Check sheet for the drawn part. Datum: minimum x, y, z corner. Units: mm. Give positions to 0.01 mm unless a question says otherwise; leave off trailing zeros. Loops run counter-clockwise (first coordinate to the right, second up) from the corner with the lowest first, then second, coordinate; pieces in that order, holes last. Notation, with made-up numbers: (-4, 48.25) - (20, 48.25) arc R22 ccw to (20, 64.25) - close; hole circle Ø10 at (0.5, 72.5). An arc over 180 degrees is marked (long way). Answer in a Markdown table with one row per item.
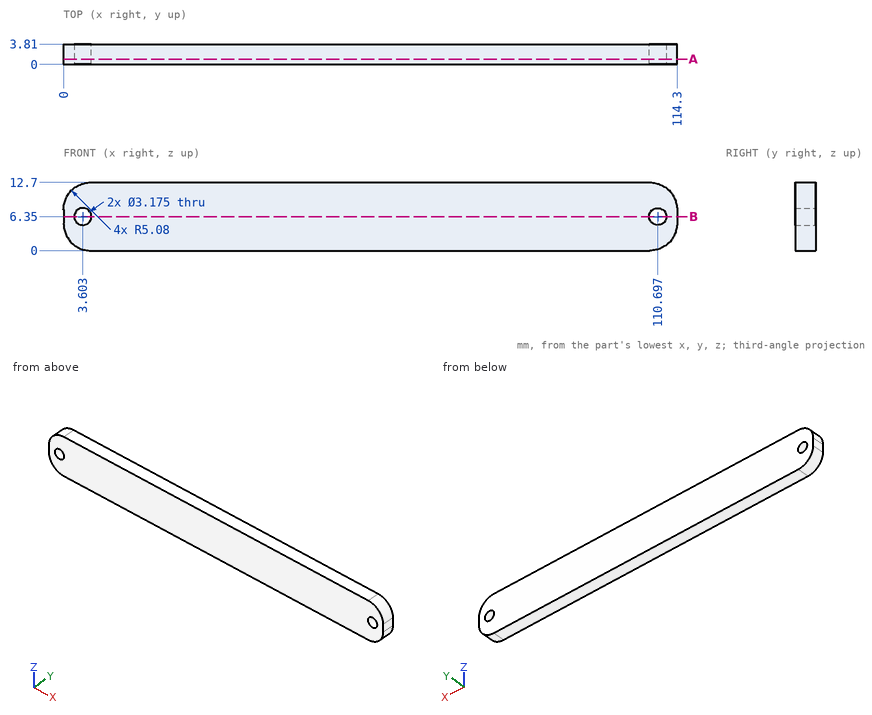
Q1. Sectioned sample at B-B (z = 6.35). Record the cut outline in (x, y), and give its area (3 significant figures).
Completed:
| item | result |
|---|---|
| outline | (0, 0) - (2.02, 0) - (2.02, 3.81) - (0, 3.81) - close; (5.19, 0) - (109.11, 0) - (109.11, 3.81) - (5.19, 3.81) - close; (112.28, 0) - (114.3, 0) - (114.3, 3.81) - (112.28, 3.81) - close |
| area | 411 mm^2 |
Q2. Thickness scan on line 1 (X direction, y = 3.3, z = 7) (1 decimal); line 2 (X direction, y = 2.1, z = 7.5); line 3 (X direction, y = 0.4, z = 4.5). Record the ranges inside material, lowest first.
Completed:
| item | result |
|---|---|
| line 1 | 0 to 2.2, 5.1 to 109.2, 112.1 to 114.3 |
| line 2 | 0 to 2.51, 4.7 to 109.6, 111.79 to 114.3 |
| line 3 | 0.03 to 114.27 |
Q3. Sectioned sample at A-A (y = 1). Give the number of separate pieces and of enclosed holes in the cut face, and give its area (3 significant figures).
Completed:
| item | result |
|---|---|
| separate pieces | 1 |
| enclosed holes | 2 |
| area | 1,410 mm^2 |
